Input: part model. Units: mm. Frame: model coordinates. A direction names the side the tool comes from. Coordinates: 2 decimals unless noted, no trailing zeros. Write each loop counter-clockwise with the first axis right and the second up, starting at its lowest first coordinate (ties: lowest second). Pieces come first, ordered by that corner, then holes. Notation, with made-up numbers: (-23.5, 49) - (-5.5, 49) arc R24 ccw to (-5.5, 80) - close; hole circle Ø10 at (-36, 88.25). An arc over 180 degrees is marked (long way). One line per question, with ' | ' between items. Start each with the question number.
1) Section query B-B on z = -16. Return loops of the section in (x, y).
2) Section query A-A on x = 37.5. Return loops of the section in (y, z), and give its area (3 significant figures).
3) Reachability of faces 4 (the cylindrical face through (-40.45, 2.03, -18.7)), 5 (the cylindrical face through (27, 5, -16)) from +Z, -Z, +X, -X, +Y, -Y: full face, straight path, thin tool, end or side. Return the list, or none.
4) Draft query along Z for faces 1 (the flat face through (-1, 3, -65)), 2 (the flat face through (-1, 3, 65)), 3 (the flat face through (37, 4, -11)). Return one class per face: released by +Z, released by -Z, zero draft, split by the parting line, or undercut.
5) First-contact query: P1, Ø5, axis at x = 37.5, z = -16, coming from the -Y side; P2, Ø13, axis at x = -37.5, z = -16, coming from the +Y side. Flat tips, straight axial feed; report the tip coordinate or a pass-through.
6) Line query: line 1 (X direction, y = 5.05, z = -16); line 2 (X direction, y = 1, z = -16); line 3 (Z direction, x = 37.5, y = 3.1). Output: solid intervals per line, ascending.
7) Section query C-C on x = -43. Return loops of the section in (y, z), and give its area (3 significant figures).
```python
from build123d import *

# Parameters (mm, degrees)
SKETCH1_W           = 100
SKETCH1_H           = 130
BOSS_EXTRUDE1_DEPTH = 6
SKETCH3_R           = 4
CUT_EXTRUDE2_DEPTH  = 7
SKETCH4_R           = 10.5
CUT_EXTRUDE3_DEPTH  = 2


with BuildPart() as part:
    # Sketch1 → Boss-Extrude1 (new body)
    with BuildSketch(Plane(origin=(0, 0, 0), x_dir=(1, 0, 0), z_dir=(0, 1, 0))):
        Rectangle(SKETCH1_W, SKETCH1_H)
    extrude(amount=BOSS_EXTRUDE1_DEPTH)

    # Sketch3 → Cut-Extrude2 (cut, through all)
    with BuildSketch(Plane(origin=(0, 6, 0), x_dir=(1, 0, 0), z_dir=(0, 1, 0))):
        with Locations((-37.5, 16)):
            Circle(SKETCH3_R)
        with Locations((37.5, 16)):
            Circle(SKETCH3_R)
    extrude(amount=-CUT_EXTRUDE2_DEPTH, mode=Mode.SUBTRACT)

    # Sketch4 → Cut-Extrude3 (cut)
    with BuildSketch(Plane(origin=(0, 6, 0), x_dir=(1, 0, 0), z_dir=(0, 1, 0))):
        with Locations((37.5, 16)):
            Circle(SKETCH4_R)
        with Locations((-37.5, 16)):
            Circle(SKETCH4_R)
    extrude(amount=-CUT_EXTRUDE3_DEPTH, mode=Mode.SUBTRACT)


solid = part.part
```
Answer key:
1) outline: (-50, 0) - (-41.5, 0) - (-41.5, 4) - (-48, 4) - (-48, 6) - (-50, 6) - close; (-33.5, 0) - (33.5, 0) - (33.5, 4) - (27, 4) - (27, 6) - (-27, 6) - (-27, 4) - (-33.5, 4) - close; (41.5, 0) - (50, 0) - (50, 6) - (48, 6) - (48, 4) - (41.5, 4) - close
2) outline: (0, -65) - (6, -65) - (6, -26.5) - (4, -26.5) - (4, -20) - (0, -20) - close; (0, -12) - (4, -12) - (4, -5.5) - (6, -5.5) - (6, 65) - (0, 65) - close | area: 706 mm²
3) face 4: +Y, -Y | face 5: +Y
4) face 1: released by -Z | face 2: released by +Z | face 3: undercut
5) P1: through | P2: y = 4
6) line 1: -50 to -48, -27 to 27, 48 to 50 | line 2: -50 to -41.5, -33.5 to 33.5, 41.5 to 50 | line 3: -65 to -20, -12 to 65
7) outline: (0, -65) - (6, -65) - (6, -24.94) - (4, -24.94) - (4, -7.06) - (6, -7.06) - (6, 65) - (0, 65) - close | area: 744 mm²
